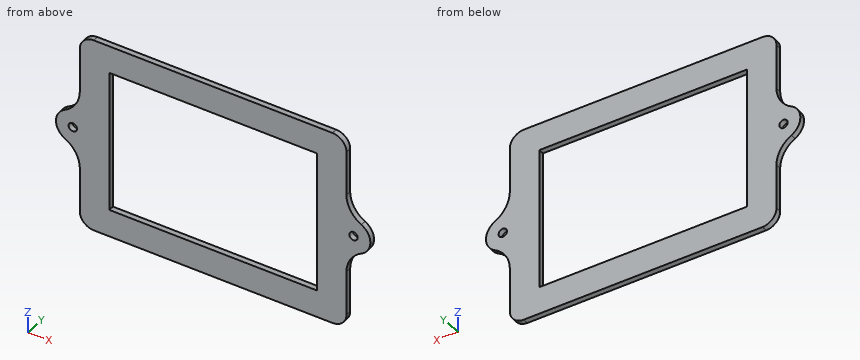
```python
from build123d import *

# Parameters (mm, degrees)
SKETCH2_R           = 1.5
SKETCH2_W           = 74
SKETCH2_H           = 50.5
BOSS_EXTRUDE1_DEPTH = 2
FILLET1_R           = 5
FILLET2_R           = 10


with BuildPart() as part:
    # Sketch2 → Boss-Extrude1 (new body)
    with BuildSketch(Plane(origin=(0, 0, 0), x_dir=(1, 0, 0), z_dir=(0, 1, 0))):
        with BuildLine():
            Line((-47.5, 35), (47.5, 35))
            Line((47.5, 35), (47.5, 5.454356057))
            ThreePointArc((47.5, 5.454356057), (56, 0), (47.5, -5.454356057))
            Line((47.5, -5.454356057), (47.5, -35))
            Line((47.5, -35), (-47.5, -35))
            Line((-47.5, -35), (-47.5, -5.454356057))
            ThreePointArc((-47.5, -5.454356057), (-56, 0), (-47.5, 5.454356057))
            Line((-47.5, 5.454356057), (-47.5, 35))
        make_face()
        with Locations(Location((-50, 0, 0), (0, 0, 270))):
            Circle(SKETCH2_R, mode=Mode.SUBTRACT)
        with Locations(Location((50, 0, 0), (0, 0, 270))):
            Circle(SKETCH2_R, mode=Mode.SUBTRACT)
        Rectangle(SKETCH2_W, SKETCH2_H, mode=Mode.SUBTRACT)
    extrude(amount=BOSS_EXTRUDE1_DEPTH)

    # Fillet1
    fillet1_edges = [part.edges().sort_by_distance(p)[0] for p in [
        (-47.5, 1, -35),
        (47.5, 1, -35),
        (47.5, 1, 35),
        (-47.5, 1, 35),
    ]]
    fillet(fillet1_edges, radius=FILLET1_R)

    # Fillet2
    fillet2_edges = [part.edges().sort_by_distance(p)[0] for p in [
        (47.5, 1, -5.454356057),
        (47.5, 1, 5.454356057),
        (-47.5, 1, 5.454356057),
        (-47.5, 1, -5.454356057),
    ]]
    fillet(fillet2_edges, radius=FILLET2_R)


solid = part.part
```
Here's how the part is built. I have some questions about the finished solid (model axes, mm). Coordinates: 2 decimals unless noted, no trailing zeros. Loops run counter-clockwise (first coordinate to the right, second up) from the corner with the lowest first, then second, coordinate; pieces in that order, holes last. Notation, with made-up numbers: (-17, -15.75) -> (21, -15.75) arc R28 ccw to (21, 7.25) -> close; hole circle Ø10 at (2.5, 67.5). An arc over 180 degrees is marked (long way). Return JSON: item names as keys, results as strings.
1) If we section it at C-C, the plane y = 1.1: Write out the boundary of the cut face in (x, z).
Results below:
{"outline": "(-52.81, -5.3) arc R10 cw to (-47.5, -14.13) -> (-47.5, -30) arc R5 ccw to (-42.5, -35) -> (42.5, -35) arc R5 ccw to (47.5, -30) -> (47.5, -14.13) arc R10 cw to (52.81, -5.3) arc R6 ccw to (52.81, 5.3) arc R10 cw to (47.5, 14.13) -> (47.5, 30) arc R5 ccw to (42.5, 35) -> (-42.5, 35) arc R5 ccw to (-47.5, 30) -> (-47.5, 14.13) arc R10 cw to (-52.81, 5.3) arc R6 ccw to start; hole circle Ø3 at (-50, 0); hole (-37, -25.25) -> (37, -25.25) -> (37, 25.25) -> (-37, 25.25) -> close; hole circle Ø3 at (50, 0)"}
2) Will these pins go through, and if not, where does the flat tip stop? pin 1 (1.8 mm diameter, centred on x = -50, z = 0, fed in from +Y); pin 2 (1 mm diameter, centred on y = 0.5, z = -18.5, fed in from +X); pin 3 (0.6 mm diameter, centred on y = 1, z = 18, fed in from -X); pin 4 (5 mm diameter, centred on x = 50, z = 0, fed in from -Y).
Results below:
{"pin 1": "through", "pin 2": "x = 47.5", "pin 3": "x = -47.5", "pin 4": "y = 0"}
3) If we section it at D-D, the plane z = 8.5: Write out the boundary of the cut face in (x, y).
Results below:
{"outline": "(-49.24, 0) -> (-37, 0) -> (-37, 2) -> (-49.24, 2) -> close; (37, 0) -> (49.24, 0) -> (49.24, 2) -> (37, 2) -> close"}
4) I need wall thicknesses on line 1 (X direction, y = 0.75, z = 0); line 2 (X direction, y = 1.7, z = -14); line 3 (Z direction, x = -36, y = 1.15). Which ranges of each line are inside material? Lowest first, please. Write a range as from..to.
Results below:
{"line 1": "-56..-51.5, -48.5..-37, 37..48.5, 51.5..56", "line 2": "-47.5..-37, 37..47.5", "line 3": "-35..-25.25, 25.25..35"}
5) If we section it at A-A, the plane z = 0: Write out the boundary of the cut face in (x, y).
Results below:
{"outline": "(-56, 0) -> (-51.5, 0) -> (-51.5, 2) -> (-56, 2) -> close; (-48.5, 0) -> (-37, 0) -> (-37, 2) -> (-48.5, 2) -> close; (37, 0) -> (48.5, 0) -> (48.5, 2) -> (37, 2) -> close; (51.5, 0) -> (56, 0) -> (56, 2) -> (51.5, 2) -> close"}
6) If we section it at B-B, the plane x = -26: Write out the boundary of the cut face in (y, z), then the cut area to 3 significant figures.
Results below:
{"outline": "(0, -35) -> (2, -35) -> (2, -25.25) -> (0, -25.25) -> close; (0, 25.25) -> (2, 25.25) -> (2, 35) -> (0, 35) -> close", "area": "39.0 mm²"}
